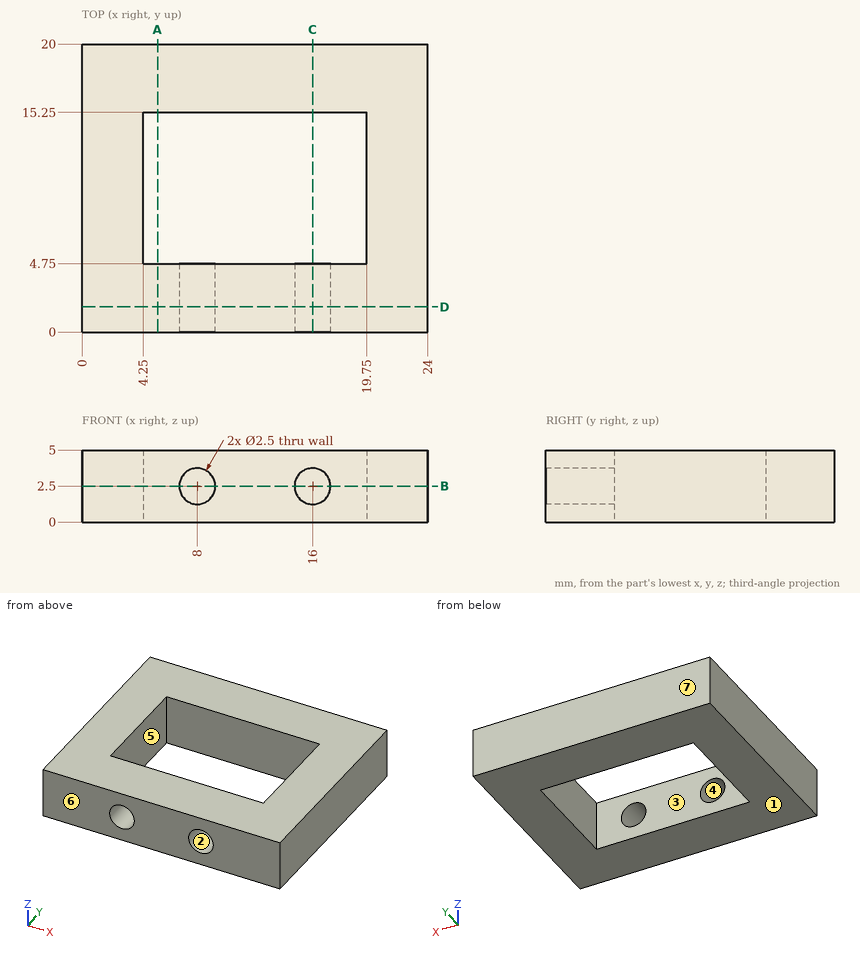
Study the drawing (mm; zero at the part's minimum x, y, z) and answer. A direction names the side the tool comes from. Give positions to 0.01 mm unless a question says otherwise; leave off trailing zeros. Write each loop counter-clockwise with the first axis right and the second up, starting at its lowest first coordinate (ties: lowest second). Pieces come first, ordered by that corner, then holes.
(1) The part is cut by section B-B on z = 2.5. Write down the section's boundary in (x, y).
Final values:
outline: (0, 0) - (6.75, 0) - (6.75, 4.75) - (4.25, 4.75) - (4.25, 15.25) - (19.75, 15.25) - (19.75, 4.75) - (17.25, 4.75) - (17.25, 0) - (24, 0) - (24, 20) - (0, 20) - close; (9.25, 0) - (14.75, 0) - (14.75, 4.75) - (9.25, 4.75) - close
(2) The part is cut by section D-D on y = 1.75. Write down the section's boundary in (x, z), plus the area to 3 significant figures.
Final values:
outline: (0, 0) - (24, 0) - (24, 5) - (0, 5) - close; hole circle Ø2.5 at (8, 2.5); hole circle Ø2.5 at (16, 2.5)
area: 110 mm2
(3) The part is cut by section A-A on x = 5.25. Write down the section's boundary in (y, z), plus the area to 3 significant figures.
Final values:
outline: (0, 0) - (4.75, 0) - (4.75, 5) - (0, 5) - close; (15.25, 0) - (20, 0) - (20, 5) - (15.25, 5) - close
area: 47.5 mm2
(4) Flat-ended cylindrical pins translate along their axes: pin 1 Ø10 at (x, y) = (14.5, 11) entering from +Z; pin 2 Ø1 at (x, y) = (10, 6.5) entering from +Z. Find the tip coordinate at first contact, or state that the pin passes through.
Final values:
pin 1: stops at z = 5
pin 2: passes through
(5) The part is cut by section C-C on x = 16. Write down the section's boundary in (y, z), plus the area to 3 significant figures.
Final values:
outline: (0, 0) - (4.75, 0) - (4.75, 1.25) - (0, 1.25) - close; (0, 3.75) - (4.75, 3.75) - (4.75, 5) - (0, 5) - close; (15.25, 0) - (20, 0) - (20, 5) - (15.25, 5) - close
area: 35.6 mm2
(6) The mould has two halves that part along Y. Classify the marked faces 4, 5, 6 and 7: pulls with the +Y half, pulls with the -Y half, needs draft (parallel to the pull), parting line crosses it, or undercut.
Final values:
face 4: needs draft
face 5: undercut
face 6: pulls with the -Y half
face 7: pulls with the +Y half
(7) Straight lines are drawn through the part: line 1 (Y direction, x = 11.5, z = 0.3); line 2 (Z direction, x = 16, y = 1.8); line 3 (X direction, y = 14.75, z = 4.35). For each, find the intervals that lie inside material, in ascending order.
Final values:
line 1: y = 0 to 4.75, 15.25 to 20
line 2: z = 0 to 1.25, 3.75 to 5
line 3: x = 0 to 4.25, 19.75 to 24
(8) Which of the six approach directions +Z, -Z, +X, -X, +Y, -Y give full straight-line access (tool end or side, diameter ignored) to the marked faces 1, 2 and 3?
Final values:
face 1: -Z, +X, -X, +Y, -Y
face 2: -Y
face 3: +Z, -Z
